from build123d import *

# Parameters (mm, degrees)
SKETCH3_R                = 4.7625
BOSS_EXTRUDE1_DEPTH      = 152.4
BOSS_EXTRUDE1_DEPTH_BACK = 152.4
CHAMFER1_SIZE            = 0.1905
SKETCH4_W                = 0.2921
SKETCH4_H                = 0.7366


with BuildPart() as part:
    # Sketch3 → Boss-Extrude1 (new body, two sides)
    with BuildSketch(Plane.XY) as boss_extrude1_sk:
        Circle(SKETCH3_R)
    extrude(amount=BOSS_EXTRUDE1_DEPTH)
    extrude(boss_extrude1_sk.sketch, amount=-BOSS_EXTRUDE1_DEPTH_BACK)

    # Chamfer1
    chamfer1_edges = [part.edges().sort_by_distance(p)[0] for p in [
        (-4.7625, 0, -152.4),
        (-4.7625, 0, 152.4),
    ]]
    chamfer(chamfer1_edges, length=CHAMFER1_SIZE)

    # Sketch4 → Cut-Revolve1 (revolve, cut)
    with BuildSketch(Plane(origin=(0, 0, 0), x_dir=(1, 0, 0), z_dir=(0, 1, 0))):
        with Locations((4.61645, 147.1683)):
            Rectangle(SKETCH4_W, SKETCH4_H)
        with Locations((4.61645, -147.1683)):
            Rectangle(SKETCH4_W, SKETCH4_H)
    revolve(axis=Axis((0, 0, 1000), (0, 0, -1)), mode=Mode.SUBTRACT)


solid = part.part
Model file for the job. Use its own axes, mm. Give positions to 0.01 mm unless a question says otherwise; leave off trailing zeros. Order: outer loops, then holes, each group sorted by start corner. A loop starts at its lowest first (then second) coordinate and runs counter-clockwise, first axis right, second up. Notation, with made-up numbers: (26, -2) - (61, -2) arc R16 ccw to (61, 21) - close; hole circle Ø10 at (45.5, -5.5). An arc over 180 degrees is marked (long way). Write item = value, one per line. Start each with the question number.
1. Cut at A-A, the plane z = -2. List the corners of the cut face in (x, y) (1 decimal).
2. Probe line 1 along X through (y, z) = (-1.25, 140); line 2 along X through (y, z) = (-0.75, 115); line 3 along Y through (x, z) = (0.5, -89). List the from-to ranges inside material, lowest first.
3. Two-plate mould, pull along Z, no slides. Class faces 1 (the flat face through (0, 0, 152.4)), 2 (the cylindrical face through (-0.969, 4.364, -147.173)), 3 (the cylindrical face through (-3.78, -2.9, 2.06)), 4 (the cylindrical face through (-0.969, 4.364, 147.163)): pulls with the +Z half, pulls with the -Z half, needs draft (parallel to the pull), parting line crosses it, or undercut.
4. Drop flat-ended pins along their axis: P1, Ø2, axis at x = -3.5, z = 73, coming from the +Y side; P2, Ø3, axis at x = -2, z = -29, coming from the -Y side; P3, Ø1, axis at x = -0.5, z = -36.5, coming from the +Y side. Give the stop position or say it passes through.
Taken from the geometry:
q1.outline = circle Ø9.5 at (0, 0)
q2.line_1 = -4.6 to 4.6
q2.line_2 = -4.7 to 4.7
q2.line_3 = -4.74 to 4.74
q3.face_1 = pulls with the +Z half
q3.face_2 = undercut
q3.face_3 = needs draft
q3.face_4 = undercut
q4.P1 = 4.05
q4.P2 = -4.74
q4.P3 = 4.76
